Geometry: see drawing. Coordinates: mm, zero at the bounding-box minimum. Coordinates: 2 decimals unless noted, no trailing zeros. Write each loop counter-clockwise with the first axis right and the second up, starting at its lowest first coordinate (ties: lowest second). Pieces come first, ordered by that corner, then holes. Notation, with made-up numbers: (45.25, 40) - (84.25, 40) arc R28 ccw to (84.25, 69) - close; hole circle Ø4 at (57, -20.75). An arc over 180 degrees is marked (long way). One line per question, with ' | ' between items. Start each with the question number.
Q1. Line query: line 1 (Y direction, x = 2.5, z = 7.75); line 2 (X direction, y = 18.5, z = 8.25); line 3 (X direction, y = 21, z = 7) (1 decimal). Output: solid intervals per line, ascending.
Q2. Cut plane B-B, the plane z = 2.25. Return loops of the section in (x, y) (1 decimal).
Q3. Cut plane D-D, the plane z = 5.5. Return loops of the section in (x, y).
Q4. Draft query along Z for the marked faces 1, 2 and 3. Return one class per face: +Z half, -Z half, draft (parallel to the pull), parting line (faces both ways), or undercut.
Q5. Cut plane C-C, the plane x = 1.5. Return loops of the section in (y, z).
Q6. Contact query for flat-ended pins moving along their axis: P1, Ø1, axis at y = 19, z = 3, coming from the -X side (1 decimal); P2, Ø6.5, axis at x = 7, z = 7, coming from the -Y side; P3, Ø8, axis at x = 3, y = 11, coming from the -Z side; P4, Ø2, axis at x = 2, y = 4.5, coming from the +Z side (1 decimal). Output: stop coordinate, or through.
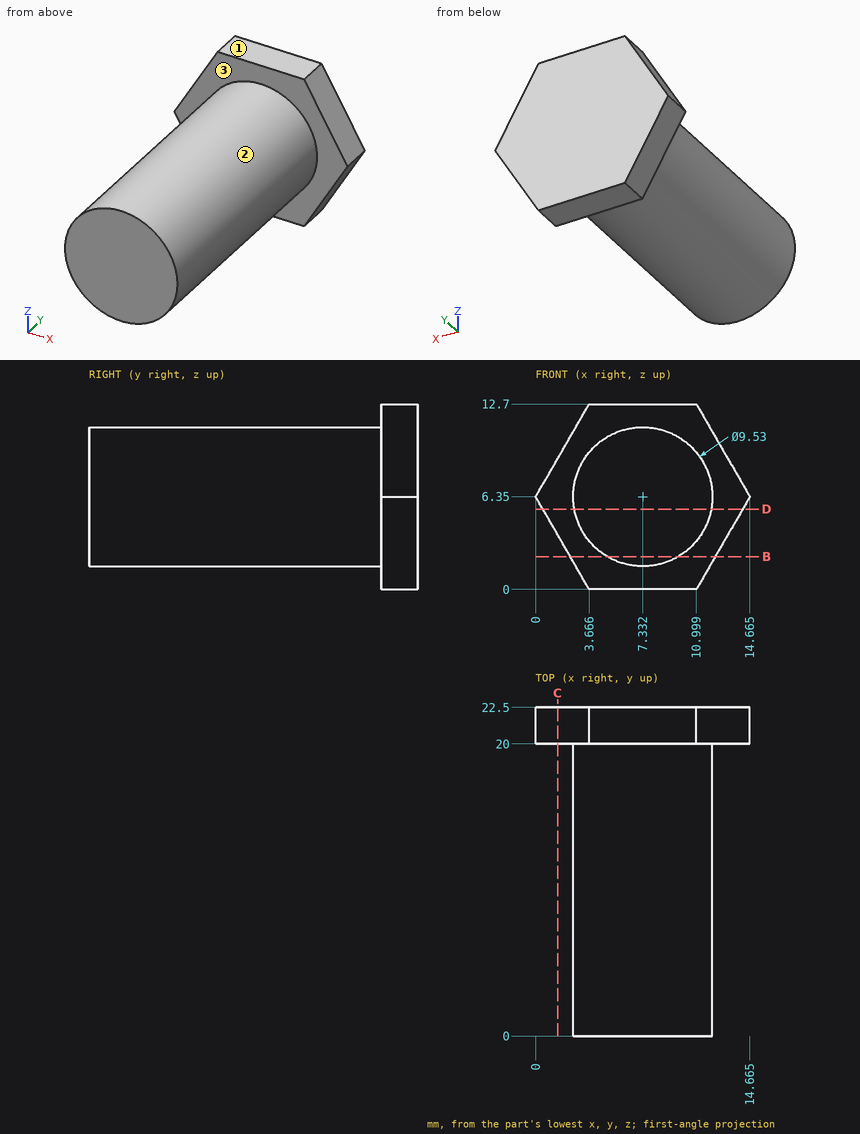
Reply:
1) line 1: y = 20 to 22.5 | line 2: x = 2.96 to 11.7 | line 3: x = 0.4 to 14.3
2) outline: (2.4, 20) - (4.9, 20) - (4.9, 0) - (9.8, 0) - (9.8, 20) - (12.3, 20) - (12.3, 22.5) - (2.4, 22.5) - close
3) outline: (0.49, 20) - (2.64, 20) - (2.64, 0) - (12.02, 0) - (12.02, 20) - (14.17, 20) - (14.17, 22.5) - (0.49, 22.5) - close
4) face 1: +Z half | face 2: parting line | face 3: draft
5) outline: (20, 3.75) - (22.5, 3.75) - (22.5, 8.95) - (20, 8.95) - close
6) P1: stops at x = 3.5 | P2: stops at y = 0 | P3: stops at z = 1.6 | P4: stops at z = 8.3
